Can you work these out from the model? Positions are in its coordinate system, mm. Coordinates: 2 decimals unless noted, no trailing zeros. Order: outer loops, then holes, each group sorted by start corner. A loop starts at its lowest first (then second) coordinate and runs counter-clockwise, first axis right, second up. Notation, with made-up numbers: (33, 55.5) -> (41, 55.5) arc R30 ccw to (41, 86.5) -> close; hole circle Ø1 at (46.25, 4.25). An arc over 180 degrees is marked (long way). Answer as CSV lines item,"result".
from build123d import *

# Parameters (mm, degrees)
SKETCH_1_W               = 72
SKETCH_1_H               = 54
EXTRUDE_1_DEPTH          = 10
CUT_EXTRUDE_1_DEPTH      = 47.097722286
CUT_EXTRUDE_1_DEPTH_BACK = 47.097722286
SKETCH_2_R               = 1.65
FILLET_1_R               = 5


with BuildPart() as part:
    # 草图1 → 凸台-拉伸1 (new body)
    with BuildSketch(Plane(origin=(0, 0, 0), x_dir=(1, 0, 0), z_dir=(0, 1, 0))):
        Rectangle(SKETCH_1_W, SKETCH_1_H)
    extrude(amount=EXTRUDE_1_DEPTH)

    # 草图2 → 切除-拉伸1 (cut, two sides: drawn at the far end of the back side and taken through both)
    with BuildSketch(Plane(origin=(0, 10, 0), x_dir=(1, 0, 0), z_dir=(0, 1, 0)).offset(-CUT_EXTRUDE_1_DEPTH_BACK)):
        with Locations(Location((-32, 16, 0), (0, 0, 270))):
            Circle(SKETCH_2_R)
        with Locations(Location((32, 16, 0), (0, 0, 270))):
            Circle(SKETCH_2_R)
        with Locations(Location((32, -16, 0), (0, 0, 270))):
            Circle(SKETCH_2_R)
        with Locations(Location((-32, -16, 0), (0, 0, 270))):
            Circle(SKETCH_2_R)
    extrude(amount=CUT_EXTRUDE_1_DEPTH + CUT_EXTRUDE_1_DEPTH_BACK, mode=Mode.SUBTRACT)

    # 圆角1
    fillet_1_edges = [part.edges().sort_by_distance(p)[0] for p in [
        (36, 5, 27),
        (-36, 5, 27),
        (-36, 5, -27),
        (36, 5, -27),
    ]]
    fillet(fillet_1_edges, radius=FILLET_1_R)


solid = part.part
Q1. Imagine slicing it at B-B (x = 32). List the corners of the cut face in (y, z) for me, and give its area (3 significant figures).
Solution:
outline,"(0, -26.9) -> (10, -26.9) -> (10, -17.65) -> (0, -17.65) -> close; (0, -14.35) -> (10, -14.35) -> (10, 14.35) -> (0, 14.35) -> close; (0, 17.65) -> (10, 17.65) -> (10, 26.9) -> (0, 26.9) -> close"
area,"472 mm2"
Q2. We'd pull the mould along X, two halves only. Please class faces 1 (the cylindrical face through (34, 5, 26)), 2 (the flat face through (0, 5, -27)), 3 (the flat face through (-36, 5, 0)), 4 (the cylindrical face through (33.39, 4.93, 16.89)): pulls with the +X half, pulls with the -X half, needs draft (parallel to the pull), parting line crosses it, or undercut.
Solution:
face 1,"pulls with the +X half"
face 2,"needs draft"
face 3,"pulls with the -X half"
face 4,"undercut"
Q3. If I drill on line 1 (X direction, y = 2.75, z = 16); line 2 (Z direction, x = 32, y = 7); line 3 (Z direction, x = 33, y = 8), over which ranges is the centre line in solid material (lowest first)?
Solution:
line 1,"-36 to -33.65, -30.35 to 30.35, 33.65 to 36"
line 2,"-26.9 to -17.65, -14.35 to 14.35, 17.65 to 26.9"
line 3,"-26.58 to -17.31, -14.69 to 14.69, 17.31 to 26.58"
Q4. Imagine slicing it at A-A (z = -16). List the corners of the cut face in (x, y) for me, and give its area (3 significant figures).
Solution:
outline,"(-36, 0) -> (-33.65, 0) -> (-33.65, 10) -> (-36, 10) -> close; (-30.35, 0) -> (30.35, 0) -> (30.35, 10) -> (-30.35, 10) -> close; (33.65, 0) -> (36, 0) -> (36, 10) -> (33.65, 10) -> close"
area,"654 mm2"
